Can you work these out from the drawing? Everything is in mm from the part's minimum corner. Round coordinates to 2 decimals unless told otherwise and drop trailing zeros. Loops run counter-clockwise (first coordinate to the right, second up) from the corner with the lowest first, then second, coordinate; pieces in that order, holes last. Notation, with made-up numbers: (39.5, -14.75) -> (96.5, -14.75) arc R19 ccw to (96.5, 12.25) -> close; hole circle Ø4 at (-2.5, 88.25). An arc over 180 degrees is marked (long way). Use CSV: the item, a comma, the result in double quotes. Start each with the question number.
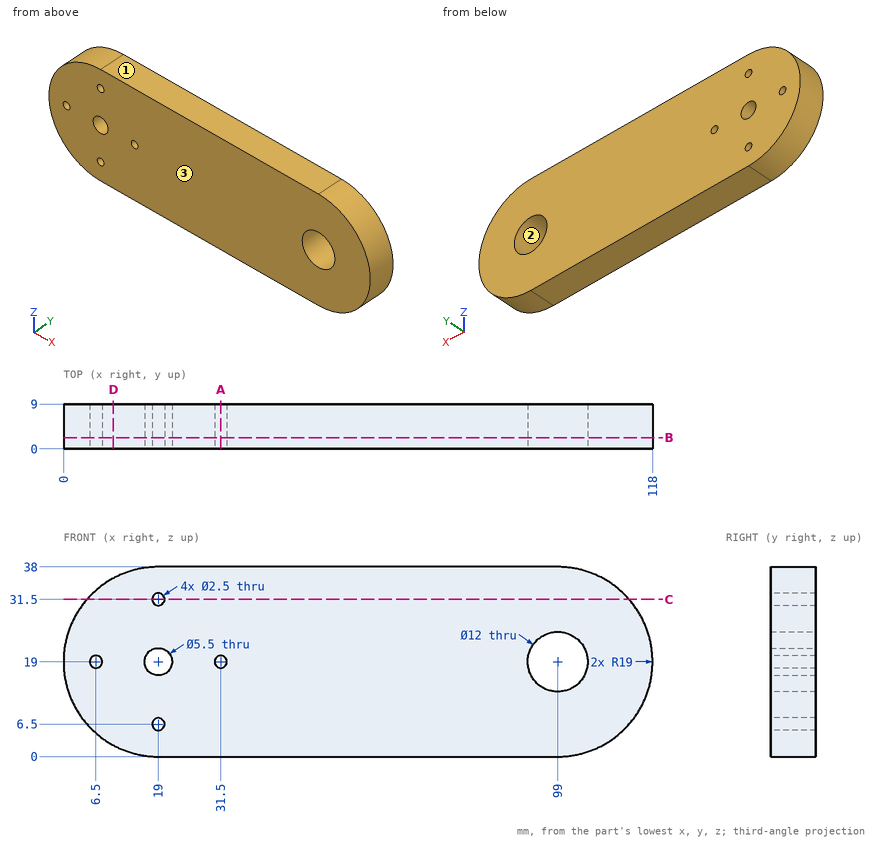
1. If I drill on L1, parallel to X at y = 3.75, z = 19; L2, parallel to X at y = 1.25, z = 18; L3, parallel to X at y = 3, z = 24.5, over which ranges is the centre line in solid material (lowest first)?
2. Suppose I cut it at A-A (x = 31.5). List the corners of the cut face in (y, z) for me.
3. Suppose I cut it at D-D (x = 10). List the corners of the cut face in (y, z) for me, then the cut area to 3 significant figures.
4. Suppose I cut it at B-B (y = 2.25). List the corners of the cut face in (x, z) for me.
5. Suppose I cut it at C-C (z = 31.5). List the corners of the cut face in (x, y) for me.
6. We'd pull the mould along Z, two halves only. Please class the marked faces 1, 2 and 3: pulls with the +Z half, pulls with the -Z half, needs draft (parallel to the pull), parting line crosses it, or undercut.
7. Will this pin go through, and if not, where does the flat tip stop? pin 1 (5 mm diameter, centred on y = 5.5, z = 6, fed in from -X).
Geometry check:
1,L1,"x = 0 to 5.25, 7.75 to 16.25, 21.75 to 30.25, 32.75 to 93, 105 to 118"
1,L2,"x = 0.03 to 5.75, 7.25 to 16.44, 21.56 to 30.75, 32.25 to 93.08, 104.92 to 117.97"
1,L3,"x = 0.81 to 96.6, 101.4 to 117.19"
2,outline,"(0, 0) -> (9, 0) -> (9, 17.75) -> (0, 17.75) -> close; (0, 20.25) -> (9, 20.25) -> (9, 38) -> (0, 38) -> close"
3,outline,"(0, 2.27) -> (9, 2.27) -> (9, 35.73) -> (0, 35.73) -> close"
3,area,"301 mm²"
4,outline,"(19, 0) -> (99, 0) arc R19 ccw to (99, 38) -> (19, 38) arc R19 ccw to start; hole circle Ø2.5 at (6.5, 19); hole circle Ø5.5 at (19, 19); hole circle Ø2.5 at (19, 6.5); hole circle Ø2.5 at (19, 31.5); hole circle Ø2.5 at (31.5, 19); hole circle Ø12 at (99, 19)"
5,outline,"(4.69, 0) -> (17.75, 0) -> (17.75, 9) -> (4.69, 9) -> close; (20.25, 0) -> (113.31, 0) -> (113.31, 9) -> (20.25, 9) -> close"
6,face 1,"pulls with the +Z half"
6,face 2,"undercut"
6,face 3,"needs draft"
7,pin 1,"stops at x = 3.16"
